Part model, mm, in its own coordinate system. Round coordinates to 2 decimals unless told otherwise and drop trailing zeros. Order: outer loops, then holes, each group sorted by start corner. A loop starts at its lowest first (then second) coordinate and runs counter-clockwise, first axis right, second up. Notation, with made-up numbers: (-21.75, 3) -> (19.25, 3) arc R20 cw to (19.25, 16) -> close; hole circle Ø3 at (1.5, 0). An arc over 180 degrees is marked (long way). Use CSV: the item, a comma, the result in double quotes.
```python
from build123d import *

# Parameters (mm, degrees)
F0_DEPTH = 180
F0_TAPER = 1
F2_DEPTH = 100
F4_T     = -2.5


with BuildPart() as f0:
    # F3 (on Top) → F0 (new body)
    with BuildSketch(Plane.XY):
        with BuildLine():
            Line((3, 15), (0, 0))
            Line((0, 0), (47, 0))
            Line((47, 0), (44, 15))
            ThreePointArc((44, 15), (23.5, 19.3957238847), (3, 15))
        make_face()
    extrude(amount=F0_DEPTH, taper=F0_TAPER)

    # F1 (on Right) → F2 (cut)
    with BuildSketch(Plane.YZ):
        Polygon((25.968901813, 3.9296671748), (0, 0), (-2.0501518156, -6.7397900857), (27.46424824, -6.7397900857), (27.54820722, -6.5070505478), align=None)
    extrude(amount=F2_DEPTH, mode=Mode.SUBTRACT)

    # F4
    f4_openings = [f0.faces().sort_by_distance(p)[0] for p in [
        (23.5, 8.769434, 1.327009),
        (23.5, 9.052127, 180),
    ]]
    offset(amount=F4_T, openings=f4_openings, kind=Kind.INTERSECTION)


solid = f0.part
```
(1) Drop flat-ended pins along their axis: P1, Ø1, axis at y = 15, z = 29, coming from the -X side; P2, Ø4, axis at y = 7.5, z = 88, coming from the -X side; P3, Ø1, axis at x = 34.5, z = 31, coming from the +Y side; P4, Ø5, axis at x = 16.5, y = 7, coming from the +Z side. Give the stop position or say it passes through.
Reply:
P1,"x = 3.42"
P2,"x = 2.66"
P3,"y = 17.73"
P4,"z = 180"
(2) Cut at A-A, the plane z = 59.5. Give the cut face in (x, y), then the cut area to 3 significant figures.
Reply:
outline,"(1.27, 1.04) -> (45.73, 1.04) -> (43.09, 14.27) arc R48.96 ccw to (3.91, 14.27) -> close; hole (4.32, 3.54) -> (42.68, 3.54) -> (40.9, 12.48) arc R46.46 ccw to (6.1, 12.48) -> close"
area,"255 mm2"
(3) Cut at B-B, the plane y = 8. Give the cut face in (x, z), then the cut area to 3 significant figures.
Reply:
outline,"(1.62, 1.21) -> (4.17, 1.21) -> (7.35, 180) -> (4.8, 180) -> close; (39.65, 180) -> (42.83, 1.21) -> (45.38, 1.21) -> (42.2, 180) -> close"
area,"912 mm2"
(4) Cut at C-C, the plane z = 151.5. Give the cut face in (x, y), then the cut area to 3 significant figures.
Reply:
outline,"(3.23, 2.64) -> (43.77, 2.64) -> (41.68, 13.12) arc R47.36 ccw to (5.32, 13.12) -> close; hole (6.28, 5.14) -> (40.72, 5.14) -> (39.49, 11.3) arc R44.86 ccw to (7.51, 11.3) -> close"
area,"224 mm2"
(5) Pull direction X, two halves, no side cores. Call faces 1 (the face through (23.786, 17.782, 92.377)), 2 (the face through (23.754, 15.285, 92.245)), 3 (the face through (23, 5, 180)): released by +X, released by -X, zero draft, split by the parting line, or undercut.
Reply:
face 1,"split by the parting line"
face 2,"undercut"
face 3,"zero draft"
(6) Probe probe 1 along Y at (x, z) = (38, 53); probe 2 along X at (y, z) = (9.5, 118); probe 3 along Y at (x, z) = (15, 29). List the from-to ranges inside material, lowest first. Write a range as [from, to].
Reply:
probe 1,"[0.93, 3.43], [13.66, 16.28]"
probe 2,"[4, 6.55], [40.45, 43]"
probe 3,"[0.51, 3.01], [15.61, 18.15]"
